from build123d import *

# Parameters (mm, degrees)
CRADLE_DEPTH                                  = 12.7
SKETCH1_R                                     = 3.175
CUT_EXTRUDE1_DEPTH                            = 12.7
QUARTER_INCH_FILLETS_R                        = 6.35
SKETCH4_R                                     = 3.175
F_0_25_28_DIAMETER_TAPPED_HOLES_FOR_LID_DEPTH = 12.7


with BuildPart() as part:
    # Base → Cradle (new body)
    with BuildSketch(Plane(origin=(0, 0, 0), x_dir=(1, 0, 0), z_dir=(0, 1, 0))):
        with BuildLine():
            Line((-27.68192265, 146.634960986), (-51.237417334, 123.079466302))
            Line((-51.237417334, 123.079466302), (-24.296648971, 96.138697939))
            Line((-24.296648971, 96.138697939), (-96.138697939, 24.296648971))
            Line((-96.138697939, 24.296648971), (-123.079466302, 51.237417334))
            Line((-123.079466302, 51.237417334), (-146.634960986, 27.68192265))
            ThreePointArc((-146.634960986, 27.68192265), (-105.518009423, 105.518009423), (-27.68192265, 146.634960986))
        make_face()
    extrude(amount=CRADLE_DEPTH)

    # Sketch1 → Cut-Extrude1 (cut)
    with BuildSketch(Plane(origin=(0, 12.7, 0), x_dir=(1, 0, 0), z_dir=(0, 1, 0))):
        with Locations((-60.217673455, 123.079466302)):
            Circle(SKETCH1_R)
        with Locations((-123.079466302, 60.217673455)):
            Circle(SKETCH1_R)
    extrude(amount=-CUT_EXTRUDE1_DEPTH, mode=Mode.SUBTRACT)

    # Quarter Inch Fillets
    quarter_inch_fillets_edges = [part.edges().sort_by_distance(p)[0] for p in [
        (-123.079466302, 6.35, -51.237417334),
        (-51.237417334, 6.35, -123.079466302),
    ]]
    fillet(quarter_inch_fillets_edges, radius=QUARTER_INCH_FILLETS_R)

    # Sketch4 → 0.25"-28 Diameter Tapped Holes for Lid (cut)
    with BuildSketch(Plane(origin=(-60.217673455, 0, -60.217673455), x_dir=(0.707106781, 0, -0.707106781), z_dir=(0.707106781, 0, 0.707106781))):
        with Locations((44.45, 6.35)):
            Circle(SKETCH4_R)
        with Locations((-44.45, 6.35)):
            Circle(SKETCH4_R)
    extrude(amount=-F_0_25_28_DIAMETER_TAPPED_HOLES_FOR_LID_DEPTH, mode=Mode.SUBTRACT)


solid = part.part
Verification items for the finished model (mm, model axes). A direction names the side the tool comes from. Coordinates: 2 decimals unless noted, no trailing zeros. Loops run counter-clockwise (first coordinate to the right, second up) from the corner with the lowest first, then second, coordinate; pieces in that order, holes last. Notation, with made-up numbers: (33, 49.5) -> (76, 49.5) arc R17 ccw to (76, 82.5) -> close; hole circle Ø5 at (-16, -27.5). An arc over 180 degrees is marked (long way). Write each question's results on one line, items separated by ' | '.
Item 1: Mould release check, pull along Z, two halves, no side actions. Record for faces 1 (the face through (-32.01, 9.03, -97.28)), 2 (the face through (-123.149, 6.439, -48.607)), 3 (the face through (-85, 0, -86)): +Z half, -Z half, draft (parallel to the pull), parting line (faces both ways), or undercut.
Found:
face 1: undercut | face 2: +Z half | face 3: draft
Item 2: Material ranges on L1, parallel to X at y = 4.5, z = -31; L2, parallel to X at y = 8.5, z = -39; L3, parallel to X at y = 2.25, z = -61, recorded low to high.
Found:
L1: x = -145.97 to -143.32, -102.84 to -97.51, -90.21 to -89.44 | L2: x = -144.04 to -135.32, -110.84 to -99.4, -98.56 to -81.44 | L3: x = -136.19 to -126.16, -120 to -59.44
Item 3: Gauge pin test, flat ends, axial feed: pin 1 (10 mm diameter, centred on x = -60.22, z = -123.08, fed in from +Y); pin 2 (6 mm diameter, centred on x = -67, y = 6.5, fed in from +Z); pin 3 (6 mm diameter, centred on x = -103, y = 2.5, fed in from -Z); pin 4 (1 mm diameter, centred on y = 2.5, z = -102.5, fed in from +X). Record the tip position at first contact, or that the pin passes through.
Found:
pin 1: stops at y = 12.7 | pin 2: stops at z = -50.44 | pin 3: stops at z = -110.76 | pin 4: stops at x = -30.16
Item 4: Section check A-A, the plane x = -42. Enter the section's corners in (y, z), plus the area to 3 significant figures.
Found:
outline: (0, -143.19) -> (12.7, -143.19) -> (12.7, -132.32) -> (0, -132.32) -> close; (0, -113.84) -> (12.7, -113.84) -> (12.7, -78.44) -> (0, -78.44) -> close | area: 588 mm2
Item 5: Section check C-C, the plane x = -105.5. Enter the section's corners in (y, z), plus the area to 3 significant figures.
Found:
outline: (0, -105.54) -> (12.7, -105.54) -> (12.7, -33.66) -> (0, -33.66) -> close | area: 913 mm2
Item 6: Tool access check on faces 4 (the face through (-37.081, 6.261, -137.236)), 5 (the face through (-37.798, 6.394, -100.597)), 6 (the face through (-136.969, 6.261, -37.348)). Record the directions out of +Z, -Z, +X, -X, +Y, -Y that give a thin tool (end or side, any length) a straight path to the whole face; none if there is none.
Found:
face 4: +X, +Y, -Y | face 5: none | face 6: +Z, +Y, -Y
Item 7: Section check B-B, the plane z = -50.5. Enter the section's corners in (x, y), plus the area to 3 significant figures.
Found:
outline: (-140.42, 0) -> (-69.94, 0) -> (-69.94, 12.7) -> (-140.42, 12.7) -> close | area: 895 mm2
